from build123d import *

# Parameters (mm, degrees)
EXTRUDE_1_DEPTH     = 27
SKETCH_2_R          = 3.25
CUT_EXTRUDE_1_DEPTH = 27
SKETCH_3_R          = 3.25
CUT_EXTRUDE_2_DEPTH = 27


with BuildPart() as part:
    # 草图1 → 凸台-拉伸1 (new body)
    with BuildSketch(Plane(origin=(0, 0, 0), x_dir=(1, 0, 0), z_dir=(0, 1, 0))):
        Polygon((0, 0), (0, 30), (-4, 30), (-4, 4), (-30, 4), (-30, 0), align=None)
    extrude(amount=EXTRUDE_1_DEPTH)

    # 草图2 → 切除-拉伸1 (cut)
    with BuildSketch(Plane(origin=(0, 0, -4), x_dir=(-1, 0, 0), z_dir=(0, 0, -1))):
        with Locations((15, 13.5)):
            Circle(SKETCH_2_R)
    extrude(amount=-CUT_EXTRUDE_1_DEPTH, mode=Mode.SUBTRACT)

    # 草图3 → 切除-拉伸2 (cut)
    with BuildSketch(Plane(origin=(0, 0, 0), x_dir=(0, 0, -1), z_dir=(1, 0, 0))):
        with Locations((15, 13.5)):
            Circle(SKETCH_3_R)
    extrude(amount=-CUT_EXTRUDE_2_DEPTH, mode=Mode.SUBTRACT)


solid = part.part
For this review, take the finished solid that the model builds, in its own axes (mm). A direction names the side the tool comes from. Give positions to 0.01 mm unless a question says otherwise; leave off trailing zeros. Loops run counter-clockwise (first coordinate to the right, second up) from the corner with the lowest first, then second, coordinate; pieces in that order, holes last. Notation, with made-up numbers: M 41.25,36 L 53.25,36 A15 ccw 53.25,44 Z; hole C 52,78.5 d4. An arc over 180 degrees is marked long. Put each result on its own line as item: value. Start each with the question number.
(1) The part is to be moulded in two halves that separate along X. For faces 3 (the cylindrical face through (-11.753, 13.643, -2.028)), 4 (the flat face through (-4, 13, -20)), 5 (the flat face through (-2, 13, -30)), 6 (the flat face through (0, 13, -11)), say which applies: +X half, -X half, draft (parallel to the pull), parting line (faces both ways), or undercut.
(2) Machinability: for faces 1 (the flat face through (-30, 13, -2)), 2 (the flat face through (-20, 13, -4)), which of the approach directions +Z, -Z, +X, -X, +Y, -Y give a long, thin tool a straight path to every point of the face, cutting with its end or side? Answer none if there is none.
(3) Wall thickness on L1, parallel to Y at x = -15, z = -2.75; L2, parallel to Z at x = -16.5, y = 3.25: over which ranges is each line inside the solid? List them lowest first.
(4) Add section D-D, the plane y = 5. Write out the cut boundary in (x, z), then the cut area to 3 significant figures.
(5) Add section B-B, the plane y = 13.5. Write out the cut boundary in (x, z), then the cut area to 3 significant figures.
(6) Add section C-C, the plane z = -15. Write out the cut boundary in (x, y), then the cut area to 3 significant figures.
(7) Add section A-A, the plane x = -15. Write out the cut boundary in (y, z).
Result:
1. face 3: undercut
1. face 4: -X half
1. face 5: draft
1. face 6: +X half
2. face 1: +Z, -Z, -X, +Y, -Y
2. face 2: -Z, -X, +Y, -Y
3. L1: y = 0 to 10.25, 16.75 to 27
3. L2: z = -4 to 0
4. outline: M -30,-4 L -4,-4 L -4,-30 L 0,-30 L 0,0 L -30,0 Z
4. area: 224 mm^2
5. outline: M -30,-4 L -18.25,-4 L -18.25,0 L -30,0 Z; M -11.75,-4 L -4,-4 L -4,-11.75 L 0,-11.75 L 0,0 L -11.75,0 Z; M -4,-30 L 0,-30 L 0,-18.25 L -4,-18.25 Z
5. area: 172 mm^2
6. outline: M -4,0 L 0,0 L 0,10.25 L -4,10.25 Z; M -4,16.75 L 0,16.75 L 0,27 L -4,27 Z
6. area: 82.0 mm^2
7. outline: M 0,-4 L 10.25,-4 L 10.25,0 L 0,0 Z; M 16.75,-4 L 27,-4 L 27,0 L 16.75,0 Z
